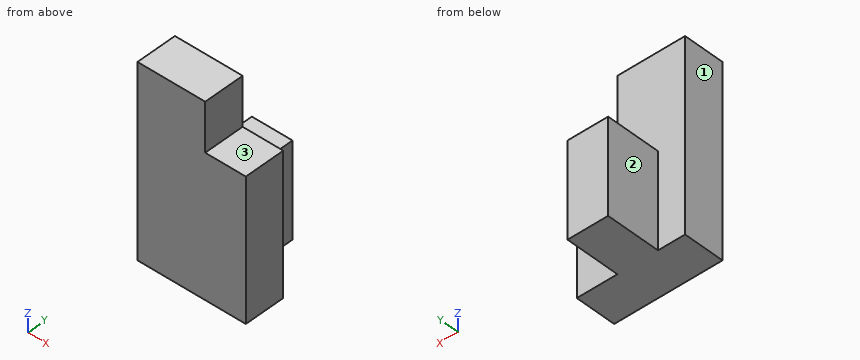
from build123d import *

# Parameters (mm, degrees)
Y_KSEKLIK_EKSTR_ZYON1_DEPTH = 15
IZIM2_W                     = 15
IZIM2_H                     = 35
Y_KSEKLIK_EKSTR_ZYON2_DEPTH = 20


with BuildPart() as part:
    # Çizim1 → Yükseklik-Ekstrüzyon1 (new body)
    with BuildSketch(Plane(origin=(0, 0, 0), x_dir=(1, 0, 0), z_dir=(0, 1, 0))):
        Polygon((5, -35), (5, -17), (20, -17), (20, 35), (-20, 35), (-20, -35), align=None)
    extrude(amount=Y_KSEKLIK_EKSTR_ZYON1_DEPTH)

    # Çizim2 → Yükseklik-Ekstrüzyon2 (add)
    with BuildSketch(Plane(origin=(0, 15, 0), x_dir=(1, 0, 0), z_dir=(0, 1, 0))):
        with Locations((-2.5, 17.5)):
            Rectangle(IZIM2_W, IZIM2_H)
    extrude(amount=Y_KSEKLIK_EKSTR_ZYON2_DEPTH)


solid = part.part
The listing builds one solid part. Answer for the finished solid, in the listing's coordinates (mm). Face numbers are marked on the shaded views. A direction names the side the tool comes from. Coordinates: 2 decimals unless noted, no trailing zeros. Loops run counter-clockwise (first coordinate to the right, second up) from the corner with the lowest first, then second, coordinate; pieces in that order, holes last. Notation, with made-up numbers: (84.5, 29.5) -> (104.5, 29.5) arc R17 ccw to (104.5, 58.5) -> close; hole circle Ø5 at (89.5, 44.25). An arc over 180 degrees is marked (long way). Answer in a Markdown table with one row per item. Add a question column.
1. For the marked faces 1, 2 and 3, determine the directions among +Z, -Z, +X, -X, +Y, -Y from which every point of the face is accessible in a straight line to the end or side of a thin tool.
2. The part is cut by section D-D, the plane y = 9. Write down the section's boundary in (x, z), then the cut area to 3 significant figures.
3. The part is cut by section A-A, the plane z = -2. Write down the section's boundary in (x, y).
4. The part is cut by section C-C, the plane y = 30. Write down the section's boundary in (x, z).
5. The part is cut by section B-B, the plane x = -5. Write down the section's boundary in (y, z).
6. Flat-ended cylindrical pins translate along their axes: P1, Ø12, axis at x = -1, y = 25, coming from the +Z side; P2, Ø1, axis at x = 16, y = 6.5, coming from the +Z side; P3, Ø6, axis at x = 10, z = 14.5, coming from the -Y side; P4, Ø10, axis at y = 29.5, z = -19.5, coming from the +X side. Find the tip coordinate at first contact, or state that the pin passes through.
7. Consider line 1 (X direction, y = 17, z = -17); line 2 (Z direction, x = 6.5, y = 2); line 3 (Y direction, x = 11.5, z = 0). Determine where each line is inside the solid, lowest interval first. Write a range as [from, to].
Answer below:
| question | item | result |
|---|---|---|
| 1 | face 1 | +Z, -Z, -X, +Y, -Y |
| 1 | face 2 | +Z, -Z, -X, +Y |
| 1 | face 3 | +Z, +X, +Y, -Y |
| 2 | outline | (-20, -35) -> (20, -35) -> (20, 17) -> (5, 17) -> (5, 35) -> (-20, 35) -> close |
| 2 | area | 2,530 mm2 |
| 3 | outline | (-20, 0) -> (20, 0) -> (20, 15) -> (5, 15) -> (5, 35) -> (-10, 35) -> (-10, 15) -> (-20, 15) -> close |
| 4 | outline | (-10, -35) -> (5, -35) -> (5, 0) -> (-10, 0) -> close |
| 5 | outline | (0, -35) -> (35, -35) -> (35, 0) -> (15, 0) -> (15, 35) -> (0, 35) -> close |
| 6 | P1 | z = 0 |
| 6 | P2 | z = 17 |
| 6 | P3 | y = 0 |
| 6 | P4 | x = 5 |
| 7 | line 1 | [-10, 5] |
| 7 | line 2 | [-35, 17] |
| 7 | line 3 | [0, 15] |
